The listing builds one solid part. Answer for the finished solid, in the listing's coordinates (mm). Face numbers are marked on the shaded views. A direction names the side the tool comes from. Round coordinates to 2 decimals unless told otherwise and drop trailing zeros. Order: outer loops, then holes, each group sorted by start corner. A loop starts at its lowest first (then second) coordinate and runs counter-clockwise, first axis right, second up. Notation, with made-up numbers: M -20.5,23.5 L 25.5,23.5 A33 cw 25.5,59.5 Z; hole C 0.5,1.25 d8. An arc over 180 degrees is marked long. Put each result on its own line as item: value. Start each with the question number.
1. Each of these flat-tipped pins is pushed along its axis until it touches: pin 1 Ø1.5 at (x, y) = (-3, 2.5) entering from +Z; pin 2 Ø1.8 at (x, z) = (5.25, -9.09) entering from -Y; pin 3 Ø1.5 at (y, z) = (6.5, 6) entering from -X; pin 4 Ø4 at (y, z) = (8.5, -7) entering from +X. Where does it stop, or does it pass through?
2. Consider line 1 (X direction, y = 0.75, z = 0); line 2 (Y direction, x = 0, z = -5) (3 decimals); line 3 (X direction, y = 14.5, z = -0.25) (3 decimals). Determine where each line is inside the solid, lowest interval first.
3. The part is cut by section C-C (y = 8.25). Give the vertices of the cut face in (x, z) (3 decimals).
4. The part is cut by section D-D (x = 4.75). Count the separate pieces of the cut face and the enclosed holes in it, then the cut area to 3 significant figures.
5. The mould has two halves that part along Z. Classify the marked faces 4, 5 and 6: +Z half, -Z half, draft (parallel to the pull), parting line (faces both ways), or undercut.
6. The part is cut by section B-B (y = 13). Give the vertices of the cut face in (x, z) (3 decimals), then the cut area to 3 significant figures.
7. Which of the six approach directions +Z, -Z, +X, -X, +Y, -Y give full straight-line access (tool end or side, diameter ignored) to the marked faces 1, 2 and 3?
from build123d import *

# Parameters (mm, degrees)
SKETCH_1_R               = 12.5
EXTRUDE_1_DEPTH          = 6
SKETCH_4_R               = 1.15
CUT_EXTRUDE_2_DEPTH      = 19
SKETCH_3_R               = 7.5
CUT_EXTRUDE_3_DEPTH      = 5
CHAMFER_2_SIZE           = 0.7
SKETCH_8_R               = 17.454292773
SKETCH_8_R_2             = 8.65
CUT_EXTRUDE_4_DEPTH      = 3
PATTERN_CIRCULAR_2_COUNT = 6
SKETCH_2_R               = 7.34982993
EXTRUDE_2_DEPTH          = 10
SKETCH_9_R               = 1.85
CUT_EXTRUDE_5_DEPTH      = 0.3
CHAMFER_3_SIZE           = 0.7
PATTERN_CIRCULAR_3_COUNT = 6
CHAMFER_4_SIZE           = 0.7
SKETCH_10_W              = 5.09
SKETCH_10_H              = 5.09
CUT_EXTRUDE_6_DEPTH      = 8.6
FILLET_1_R               = 2
CHAMFER_5_SIZE           = 5.09


# Some blends are built 0.0001 mm under size
with BuildPart() as part:
    # 草图1 → 凸台-拉伸1 (new body)
    with BuildSketch(Plane(origin=(0, 0, 0), x_dir=(1, 0, 0), z_dir=(0, 1, 0))):
        with Locations(Location((0, 0, 0), (0, 0, 270))):
            Circle(SKETCH_1_R)
    extrude(amount=EXTRUDE_1_DEPTH)

    # 草图4 → 切除-拉伸2 (cut)
    with BuildSketch(Plane(origin=(0, 6, 0), x_dir=(1, 0, 0), z_dir=(0, 1, 0))):
        with Locations(Location((-10.5, 0, 0), (0, 0, 270))):
            Circle(SKETCH_4_R)
    cut_extrude_2 = extrude(amount=-CUT_EXTRUDE_2_DEPTH, mode=Mode.SUBTRACT)

    # 草图3 → 切除-拉伸3 (cut)
    with BuildSketch(Plane(origin=(0, 0, 0), x_dir=(-1, 0, 0), z_dir=(0, -1, 0))):
        with Locations(Location((0, 0, 0), (0, 0, 90))):
            Circle(SKETCH_3_R)
    extrude(amount=-CUT_EXTRUDE_3_DEPTH, mode=Mode.SUBTRACT)

    # 倒角2
    chamfer_2_edges = [part.edges().sort_by_distance(p)[0] for p in [
        (-10.5, 6, -1.15),
    ]]
    chamfer(chamfer_2_edges, length=CHAMFER_2_SIZE)

    # 草图8 → 切除-拉伸4 (cut)
    with BuildSketch(Plane(origin=(0, 6, 0), x_dir=(1, 0, 0), z_dir=(0, 1, 0))):
        Circle(SKETCH_8_R)
        with Locations(Location((0, 0, 0), (0, 0, 270))):
            Circle(SKETCH_8_R_2, mode=Mode.SUBTRACT)
    extrude(amount=-CUT_EXTRUDE_4_DEPTH, mode=Mode.SUBTRACT)

    # 阵列(圆周)2: 切除-拉伸2 ×6 about axis
    pattern_circular_2_axis = Axis((0, 0, 0), (0, 1, 0))
    for i in range(1, PATTERN_CIRCULAR_2_COUNT):
        add(cut_extrude_2.rotate(pattern_circular_2_axis, i * 360 / PATTERN_CIRCULAR_2_COUNT), mode=Mode.SUBTRACT)

    # 草图2 → 凸台-拉伸2 (add)
    with BuildSketch(Plane(origin=(0, 6, 0), x_dir=(1, 0, 0), z_dir=(0, 1, 0))):
        with Locations(Location((0, 0, 0), (0, 0, 270))):
            Circle(SKETCH_2_R)
    extrude(amount=EXTRUDE_2_DEPTH)

    # 草图9 → 切除-拉伸5 (cut)
    with BuildSketch(Plane(origin=(0, 3, 0), x_dir=(1, 0, 0), z_dir=(0, 1, 0))):
        with Locations(Location((-10.5, 0, 0), (0, 0, 270))):
            Circle(SKETCH_9_R)
    cut_extrude_5 = extrude(amount=-CUT_EXTRUDE_5_DEPTH, mode=Mode.SUBTRACT)

    # 倒角3
    chamfer_3_edges = [part.edges().sort_by_distance(p)[0] for p in [
        (-10.5, 2.7, -1.15),
    ]]
    chamfer(chamfer_3_edges, length=CHAMFER_3_SIZE - 0.0001)  # a hair under: the kernel refuses the full size

    # 阵列(圆周)3: 切除-拉伸5 ×6 about axis
    pattern_circular_3_axis = Axis((0, 0, 0), (0, 1, 0))
    for i in range(1, PATTERN_CIRCULAR_3_COUNT):
        add(cut_extrude_5.rotate(pattern_circular_3_axis, i * 360 / PATTERN_CIRCULAR_3_COUNT), mode=Mode.SUBTRACT)

    # 倒角4
    chamfer_4_edges = [part.edges().sort_by_distance(p)[0] for p in [
        (-4.254070786, 2.7, -9.66826674),
        (6.245929214, 2.7, -8.51826674),
        (10.5, 2.7, 1.15),
        (4.254070786, 2.7, 9.66826674),
        (-6.245929214, 2.7, 8.51826674),
    ]]
    chamfer(chamfer_4_edges, length=CHAMFER_4_SIZE - 0.0001)  # a hair under: the kernel refuses the full size

    # 草图10 → 切除-拉伸6 (cut)
    with BuildSketch(Plane(origin=(0, 16, 0), x_dir=(1, 0, 0), z_dir=(0, 1, 0))):
        Rectangle(SKETCH_10_W, SKETCH_10_H)
    extrude(amount=-CUT_EXTRUDE_6_DEPTH, mode=Mode.SUBTRACT)

    # 草图11 → 切除-旋转1 (revolve, cut)
    with BuildSketch(Plane(origin=(0, 0, 0), x_dir=(0, 0, -1), z_dir=(1, 0, 0)), mode=Mode.PRIVATE) as cut_revolve_1_sk:
        Polygon((-0.304897272, 10.075), (-10.874100718, 10.075), (-10.874100718, 6), (-4.145, 6), (-4.145, 7.875), (-2.545, 7.875), (-2.545, 9.125), (11.125701635, 9.125), (11.125701635, 10.075), align=None)
    revolve(cut_revolve_1_sk.sketch.rotate(Axis((0, 10.075, 0.304897272), (0, 0, 1)), 180), axis=Axis((0, 10.075, 0.304897272), (0, 0, 1)), mode=Mode.SUBTRACT)

    # 圆角1
    # the kernel refuses this fillet: 2 mm, written as the material it takes off along each edge
    with BuildSketch(Plane(origin=(0, 16, 0), x_dir=(0, 0, 1), z_dir=(-1, 0, 0))) as fillet_1_piece_1:
        with BuildLine():
            CenterArc((7.34982993 - FILLET_1_R, -FILLET_1_R), FILLET_1_R, 0, 90)
            Line((7.34982993 - FILLET_1_R, 0), (7.34982993, 0))
            Line((7.34982993, 0), (7.34982993, -FILLET_1_R))
        make_face()
    revolve(axis=Axis((0, 16, 0), (0, 1, 0)), mode=Mode.SUBTRACT)

    # 倒角5
    # the kernel refuses this chamfer: 5.09 mm, written as the material it adds along each edge
    with BuildSketch(Plane(origin=(2.545, 7.4, -2.545), x_dir=(0, 0.9996219169112968, -0.027495876610586393), z_dir=(-1, 0, 0))) as chamfer_5_piece_1_section:
        Polygon((CHAMFER_5_SIZE * 0.999621916911, -CHAMFER_5_SIZE * 0.0274958766106), (-CHAMFER_5_SIZE * 0.0274958766106, -CHAMFER_5_SIZE * 0.999621916911), (0, 0), align=None)
    chamfer_5_piece_1 = extrude(amount=5.09, mode=Mode.PRIVATE)
    chamfer_5_piece_1 = chamfer_5_piece_1 - Plane(origin=(0, 10.075, -0.813981716), x_dir=(0, 1, 0), z_dir=(0, 0, -1)) * Cylinder(0.95, 31, mode=Mode.PRIVATE)
    add(chamfer_5_piece_1)


solid = part.part
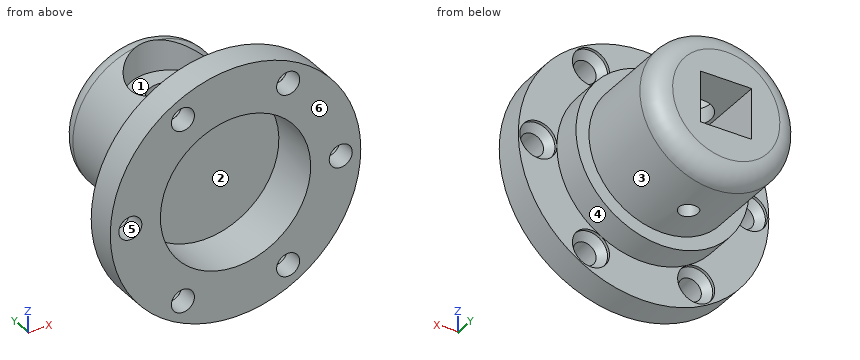
Resolved:
1. pin 1: z = 12.3
1. pin 2: through
1. pin 3: x = -6.72
1. pin 4: x = 5.39
2. line 1: -12.5 to -11.65, -9.35 to -7.5, 7.5 to 9.35, 11.65 to 12.5
2. line 2: 5 to 9.125, 11.025 to 16
2. line 3: -7.282 to -2.545, 2.545 to 7.282
3. outline: M -3.643,4.145 L -3.643,6.383 A7.35 ccw long 3.643,6.383 L 3.643,4.145 L 1.229,4.145 L 1.229,2.545 L 2.545,2.545 L 2.545,1.695 L -2.545,1.695 L -2.545,2.545 L -1.229,2.545 L -1.229,4.145 Z
4. separate pieces: 3
4. enclosed holes: 0
4. area: 150 mm2
5. face 4: parting line
5. face 5: undercut
5. face 6: draft
6. outline: M -2.837,4.145 L -2.837,6.78 A7.35 ccw long 2.837,6.78 L 2.837,4.145 Z; hole M -2.545,-2.545 L 2.545,-2.545 L 2.545,2.545 L -2.545,2.545 Z
6. area: 127 mm2
7. face 1: +Z
7. face 2: -Y
7. face 3: +Y
